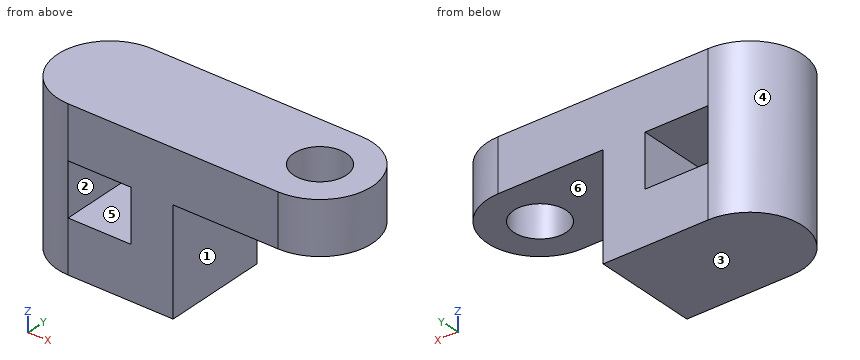
from build123d import *

# Parameters (mm, degrees)
SKETCH2_R                = 2.5
BOSS_EXTRUDE1_DEPTH      = 5
BOSS_EXTRUDE2_DEPTH      = 10
BOSS_EXTRUDE2_DEPTH_BACK = 5
SKETCH4_W                = 6
SKETCH4_H                = 5
CUT_EXTRUDE1_DEPTH       = 10


with BuildPart() as part:
    # Sketch2 → Boss-Extrude1 (new body)
    with BuildSketch(Plane.XY):
        with BuildLine():
            Line((0, 5), (20, 5))
            ThreePointArc((20, 5), (25, 0), (20, -5))
            Line((20, -5), (0, -5))
            ThreePointArc((0, -5), (-5, 0), (0, 5))
        make_face()
        with Locations((20, 0)):
            Circle(SKETCH2_R, mode=Mode.SUBTRACT)
    extrude(amount=BOSS_EXTRUDE1_DEPTH)

    # Sketch3 → Boss-Extrude2 (add, two sides: drawn at the far end of the back side and taken through both)
    with BuildSketch(Plane(origin=(0, 0, 0), x_dir=(-1, 0, 0), z_dir=(0, 0, -1)).offset(-BOSS_EXTRUDE2_DEPTH_BACK)):
        with BuildLine():
            Line((-10, 5), (0, 5))
            ThreePointArc((0, 5), (5, 0), (0, -5))
            Line((0, -5), (-10, -5))
            Line((-10, -5), (-10, 5))
        make_face()
    extrude(amount=BOSS_EXTRUDE2_DEPTH + BOSS_EXTRUDE2_DEPTH_BACK)

    # Sketch4 → Cut-Extrude1 (cut)
    with BuildSketch(Plane(origin=(0, 5, 0), x_dir=(1, 0, 0), z_dir=(0, 1, 0))):
        with Locations((3, 2.5)):
            Rectangle(SKETCH4_W, SKETCH4_H)
    extrude(amount=-CUT_EXTRUDE1_DEPTH, mode=Mode.SUBTRACT)


solid = part.part
Work out the finished part from the listing and answer in its coordinate system (mm). Face numbers are marked on the shaded views. A direction names the side the tool comes from. Give positions to 0.01 mm unless a question says otherwise; leave off trailing zeros. Write each loop counter-clockwise with the first axis right and the second up, starting at its lowest first coordinate (ties: lowest second). Pieces come first, ordered by that corner, then holes.
Q1. Given pin 1 (4 mm diameter, centred on x = 20, y = 0, fed in from +Z); pin 2 (1.5 mm diameter, centred on y = -0.5, z = -3.5, fed in from +X); pin 3 (1.5 mm diameter, centred on y = 2.5, z = -6.5, fed in from -X); pin 4 (6 mm diameter, centred on x = 21.5, y = -2.5, fed in from -Z), each flat-ended and moving along its own axis, determine where each tip first touches the part or whether it passes through.
Answer:
pin 1: passes through
pin 2: stops at x = 10
pin 3: stops at x = -4.68
pin 4: stops at z = 0
Q2. The part is cut by section D-D on z = 3. Give the vertices of the cut face in (x, y), and give its area (3 significant figures).
Answer:
outline: (0, -5) - (20, -5) arc R5 ccw to (20, 5) - (0, 5) arc R5 ccw to start; hole circle Ø5 at (20, 0)
area: 259 mm2
Q3. The part is cut by section B-B on z = -3.25. Give the vertices of the cut face in (x, y).
Answer:
outline: (0, -5) - (0, 5) arc R5 ccw to start; (6, -5) - (10, -5) - (10, 5) - (6, 5) - close
Q4. For a pull along X with two mould halves and no side action, classify the marked faces 1, 2 and 3 as released by +X, released by -X, zero draft, split by the parting line, or undercut.
Answer:
face 1: released by +X
face 2: undercut
face 3: zero draft
Q5. A tool of negligible diameter and unlimited length cuts with its end or side. For the marked faces 4, 5 and 6, from which of +Z, -Z, +X, -X, +Y, -Y can it reach the whole face along a straight path? Write none if from no direction.
Answer:
face 4: +Z, -Z, -X
face 5: +Y, -Y
face 6: -Z, +X, +Y, -Y
Q6. The part is cut by section C-C on x = 4.5. Give the vertices of the cut face in (y, z), and give its area (3 significant figures).
Answer:
outline: (-5, -10) - (5, -10) - (5, -5) - (-5, -5) - close; (-5, 0) - (5, 0) - (5, 5) - (-5, 5) - close
area: 100 mm2
Q7. Straight lines are drawn through the part: L1, parallel to Y at x = 20, z = 1.3; L2, parallel to Z at x = 5, y = -2.5; L3, parallel to Z at x = 15.75, y = -0.25. For each, find the intervals that lie inside material, in ascending order.
Answer:
L1: y = -5 to -2.5, 2.5 to 5
L2: z = -10 to -5, 0 to 5
L3: z = 0 to 5
Q8. The part is cut by section A-A on y = 0. Give the vertices of the cut face in (x, z), and give its area (3 significant figures).
Answer:
outline: (-5, -10) - (10, -10) - (10, 0) - (17.5, 0) - (17.5, 5) - (-5, 5) - close; (22.5, 0) - (25, 0) - (25, 5) - (22.5, 5) - close; hole (0, -5) - (6, -5) - (6, 0) - (0, 0) - close
area: 245 mm2
